Read the model definition and answer for the solid it produces. Units are mm, in the model's axes. Face numbers are marked on the shaded views. Coordinates: 2 decimals unless noted, no trailing zeros. Write each loop counter-clockwise with the first axis right and the second up, starting at its lowest first coordinate (ties: lowest second). Pieces come first, ordered by that corner, then holes.
1) Find the intervals of material crossed by line 1 (Y direction, x = 30.75, z = -158); line 2 (Y direction, x = 13, z = -12.5); line 3 (Z direction, x = 11.75, y = 55.5), in increasing order.
2) The part is cut by section B-B (x = 29.5). Determine the outline of the cut face in (y, z), then the cut area to 3 significant figures.
3) Each of these flat-tipped pins is pushed along its axis until it touches: pin 1 Ø3 at (x, z) = (10.5, -44) entering from +Y; pin 2 Ø12 at (x, z) = (10, -6.5) entering from -Y; pin 3 Ø5 at (x, y) = (10, 10) entering from -Z; pin 4 Ø4.5 at (y, z) = (-76, 133) entering from +X. Where does it stop, or does it pass through?
4) The part is cut by section C-C (z = 17.5). Determine the outline of the cut face in (x, y), then the cut area to 3 significant figures.
5) Determine the mould class of the marked faces 1 and 2 for opening direction Z: +Z half, -Z half, draft (parallel to the pull), parting line (faces both ways), or undercut.
6) The part is cut by section A-A (y = 0). Determine the outline of the cut face in (x, z).
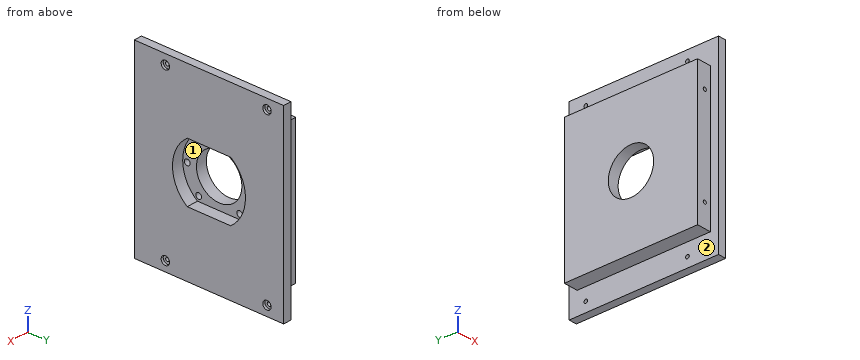
from build123d import *

# Parameters (mm, degrees)
SKETCH1_W                               = 325
SKETCH1_H                               = 260
BOSS_EXTRUDE1_DEPTH                     = 39
CBORE_FOR_M6_HEX_HEAD_BOLT1_D           = 6.4
CBORE_FOR_M6_HEX_HEAD_BOLT1_DEPTH       = 30
CBORE_FOR_M6_HEX_HEAD_BOLT1_CBORE_D     = 14.547
CBORE_FOR_M6_HEX_HEAD_BOLT1_CBORE_DEPTH = 4
CBORE_FOR_M6_HEX_HEAD_BOLT1_TIP         = 1.922753981
SKETCH3_R                               = 39.51
CUT_EXTRUDE2_DEPTH                      = 39
CUT_EXTRUDE3_DEPTH                      = 19.8
F_10_0MM_DOWEL_HOLE1_D                  = 10
F_10_0MM_DOWEL_HOLE1_DEPTH              = 30
F_10_0MM_DOWEL_HOLE1_TIP                = 3.004303095
SKETCH18_W                              = 39
SKETCH18_H                              = 260
CUT_EXTRUDE5_DEPTH                      = 25
SKETCH19_W                              = 25
SKETCH19_H                              = 247
CUT_EXTRUDE6_DEPTH                      = 14
F_6_0MM_DOWEL_HOLE1_D                   = 6
F_6_0MM_DOWEL_HOLE1_DEPTH               = 15
F_6_0MM_DOWEL_HOLE1_TIP                 = 1.802581857
CUT_EXTRUDE7_DEPTH                      = 222.463315247
CUT_EXTRUDE7_DEPTH_BACK                 = 222.463315247
SKETCH23_W                              = 25
SKETCH23_H                              = 14


with BuildPart() as part:
    # Sketch1 → Boss-Extrude1 (new body)
    with BuildSketch(Plane(origin=(0, 0, 0), x_dir=(0, 0, -1), z_dir=(1, 0, 0))):
        with Locations((12.5, 0)):
            Rectangle(SKETCH1_W, SKETCH1_H)
    extrude(amount=BOSS_EXTRUDE1_DEPTH)

    # CBORE for M6 Hex Head Bolt1
    with Locations(Plane(origin=(39, 0, 0), x_dir=(0, 0, -1), z_dir=(1, 0, 0))):
        with Locations((158, 101), (158, -76), (-133, 101), (-133, -76)):
            CounterBoreHole(CBORE_FOR_M6_HEX_HEAD_BOLT1_D / 2, CBORE_FOR_M6_HEX_HEAD_BOLT1_CBORE_D / 2, CBORE_FOR_M6_HEX_HEAD_BOLT1_CBORE_DEPTH, depth=CBORE_FOR_M6_HEX_HEAD_BOLT1_DEPTH)
            with Locations((0, 0, -(CBORE_FOR_M6_HEX_HEAD_BOLT1_DEPTH + CBORE_FOR_M6_HEX_HEAD_BOLT1_TIP / 2))):  # 118° drill point
                Cone(0, CBORE_FOR_M6_HEX_HEAD_BOLT1_D / 2, CBORE_FOR_M6_HEX_HEAD_BOLT1_TIP, mode=Mode.SUBTRACT)

    # Sketch3 → Cut-Extrude2 (cut)
    with BuildSketch(Plane(origin=(39, 0, 0), x_dir=(0, 0, -1), z_dir=(1, 0, 0))):
        with Locations((12.5, 0)):
            Circle(SKETCH3_R)
    extrude(amount=-CUT_EXTRUDE2_DEPTH, mode=Mode.SUBTRACT)

    # Sketch5 → Cut-Extrude3 (cut)
    with BuildSketch(Plane(origin=(39, 0, 0), x_dir=(0, 0, -1), z_dir=(1, 0, 0))):
        with BuildLine():
            Line((-38.5, 37.85), (-38.5, -37.85))
            ThreePointArc((-38.5, -37.85), (12.5, -63.518135124), (63.5, -37.85))
            Line((63.5, -37.85), (63.5, 37.85))
            ThreePointArc((63.5, 37.85), (12.5, 63.518135124), (-38.5, 37.85))
        make_face()
    extrude(amount=-CUT_EXTRUDE3_DEPTH, mode=Mode.SUBTRACT)

    # Ø10.0mm Dowel Hole1
    with Locations(Plane(origin=(39, 0, 0), x_dir=(0, 0, -1), z_dir=(1, 0, 0))):
        with Locations((12.5, 55.5), (55.015466593, 35.674712338), (-30.015466593, 35.674712338), (-30.015466593, -35.674712338), (12.5, -55.5), (55.015466593, -35.674712338)):
            Hole(F_10_0MM_DOWEL_HOLE1_D / 2, depth=F_10_0MM_DOWEL_HOLE1_DEPTH)
            with Locations((0, 0, -(F_10_0MM_DOWEL_HOLE1_DEPTH + F_10_0MM_DOWEL_HOLE1_TIP / 2))):  # 118° drill point
                Cone(0, F_10_0MM_DOWEL_HOLE1_D / 2, F_10_0MM_DOWEL_HOLE1_TIP, mode=Mode.SUBTRACT)

    # Sketch18 → Cut-Extrude5 (cut)
    with BuildSketch(Plane(origin=(0, 0, 0), x_dir=(0, 0, -1), z_dir=(1, 0, 0))):
        with Locations((155.5, 0)):
            Rectangle(SKETCH18_W, SKETCH18_H)
        with Locations((-130.5, 0)):
            Rectangle(SKETCH18_W, SKETCH18_H)
    extrude(amount=CUT_EXTRUDE5_DEPTH, mode=Mode.SUBTRACT)

    # Sketch19 → Cut-Extrude6 (cut)
    with BuildSketch(Plane(origin=(0, -130, 0), x_dir=(-1, 0, 0), z_dir=(0, -1, 0))):
        with Locations((-12.5, 12.5)):
            Rectangle(SKETCH19_W, SKETCH19_H)
    extrude(amount=-CUT_EXTRUDE6_DEPTH, mode=Mode.SUBTRACT)

    # Ø6.0mm Dowel Hole1
    with Locations(Plane(origin=(0, -116, 0), x_dir=(-1, 0, 0), z_dir=(0, -1, 0))):
        with Locations((-14, 96.5), (-14, -71.5)):
            Hole(F_6_0MM_DOWEL_HOLE1_D / 2, depth=F_6_0MM_DOWEL_HOLE1_DEPTH)
            with Locations((0, 0, -(F_6_0MM_DOWEL_HOLE1_DEPTH + F_6_0MM_DOWEL_HOLE1_TIP / 2))):  # 118° drill point
                Cone(0, F_6_0MM_DOWEL_HOLE1_D / 2, F_6_0MM_DOWEL_HOLE1_TIP, mode=Mode.SUBTRACT)

    # Sketch23 → Cut-Extrude7 (cut, two sides: drawn at the far end of the back side and taken through both)
    with BuildSketch(Plane.XY.offset(-CUT_EXTRUDE7_DEPTH_BACK)):
        with Locations((12.5, 123)):
            Rectangle(SKETCH23_W, SKETCH23_H)
    extrude(amount=CUT_EXTRUDE7_DEPTH + CUT_EXTRUDE7_DEPTH_BACK, mode=Mode.SUBTRACT)


solid = part.part
Reported:
1. line 1: y = -130 to -79.2, -72.8 to 97.8, 104.2 to 130
1. line 2: y = -116 to -60.5, -50.5 to -39.51, 39.51 to 50.5, 60.5 to 116
1. line 3: z = -136 to -17.5, -7.5 to 111
2. outline: (-130, -175) - (130, -175) - (130, 150) - (-130, 150) - close; hole circle Ø6.4 at (-76, -158); hole circle Ø6.4 at (-76, 133); hole (-37.85, -63.5) - (37.85, -63.5) arc R63.5 ccw to (37.85, 38.5) - (-37.85, 38.5) arc R63.5 ccw to start; hole circle Ø6.4 at (101, -158); hole circle Ø6.4 at (101, 133)
2. area: 73,000 mm2
3. pin 1: stops at y = 116
3. pin 2: stops at y = -116
3. pin 3: stops at z = -136
3. pin 4: passes through
4. outline: (0, -116) - (25, -116) - (25, -130) - (39, -130) - (39, -55.98) - (19.2, -55.98) - (19.2, -25.71) - (0, -25.71) - close; (0, 25.71) - (19.2, 25.71) - (19.2, 55.98) - (39, 55.98) - (39, 130) - (25, 130) - (25, 116) - (0, 116) - close
4. area: 6,240 mm2
5. face 1: undercut
5. face 2: draft
6. outline: (0, -136) - (25, -136) - (25, -175) - (39, -175) - (39, -63.5) - (19.2, -63.5) - (19.2, -52.01) - (0, -52.01) - close; (0, 27.01) - (19.2, 27.01) - (19.2, 38.5) - (39, 38.5) - (39, 150) - (25, 150) - (25, 111) - (0, 111) - close
